from build123d import *

# Parameters (mm, degrees)
SKETCH_1_W          = 12
SKETCH_1_H          = 28
EXTRUDE_1_DEPTH     = 2
SKETCH_2_W          = 12
SKETCH_2_H          = 17
EXTRUDE_2_DEPTH     = 5
CUT_EXTRUDE_1_REACH = 18.031
SKETCH_3_R          = 1


with BuildPart() as part:
    # 草图1 → 凸台-拉伸1 (new body)
    with BuildSketch(Plane.XY):
        Rectangle(SKETCH_1_W, SKETCH_1_H)
    extrude(amount=-EXTRUDE_1_DEPTH)

    # 草图2 → 凸台-拉伸2 (add)
    with BuildSketch(Plane.XY):
        with Locations((0, 5.5)):
            Rectangle(SKETCH_2_W, SKETCH_2_H)
    extrude(amount=EXTRUDE_2_DEPTH)

    # 草图3 → 切除-拉伸1 (cut, up to next)
    with BuildSketch(Plane.XY, mode=Mode.PRIVATE) as cut_extrude_1_sk1:
        with Locations((0, -8)):
            Circle(SKETCH_3_R)
    cut_extrude_1_tool1 = extrude(cut_extrude_1_sk1.sketch, amount=-CUT_EXTRUDE_1_REACH, mode=Mode.PRIVATE) & part.part
    add(cut_extrude_1_tool1.solids().sort_by_distance((0, -8, 0))[0], mode=Mode.SUBTRACT)


solid = part.part
Here's how the part is built. I have some questions about the finished solid (model axes, mm). A direction names the side the tool comes from. Give positions to 0.01 mm unless a question says otherwise; leave off trailing zeros. Order: outer loops, then holes, each group sorted by start corner. A loop starts at its lowest first (then second) coordinate and runs counter-clockwise, first axis right, second up. Notation, with made-up numbers: (-6.75, -2) -> (49.25, -2) arc R16 cw to (49.25, 21) -> close; hole circle Ø11 at (26.5, 20). An arc over 180 degrees is marked (long way). Use a Markdown table: item, result. Add a question column.
Item 1: Imagine slicing it at B-B on x = 0. Please give me the cut outline in (y, z).
Item 2: Imagine slicing it at A-A on y = -8. Please give me the cut outline in (x, z), plus the area to 3 significant figures.
Item 3: Imagine slicing it at C-C on x = 4. Please give me the cut outline in (y, z).
Item 4: I need wall thicknesses on line 1 (Y direction, x = 0, z = -1); line 2 (Z direction, x = 3.25, y = -7.5); line 3 (Y direction, x = -3.75, z = 1.25). Which ranges of each line are inside material? Lowest first, please.
Item 5: Imagine slicing it at D-D on z = 2. Please give me the cut outline in (x, y).
Item 6: For faces 1 (the face through (0, -14, -1)), 2 (the face through (0, -10, 0)), which set-ups out of +Z, -Z, +X, -X, +Y, -Y let a thin tool reach every point of the face, with its end or its side?
Item 7: If we mould it in two halves opening along Y, with no side actions, what happens to faces 3 (the face through (0, 14, 1)), 4 (the face through (0, -3, 2)), 5 (the face through (0, 6, 5)), 6 (the face through (0, -7, -1))? For each: pulls with the +Y half, pulls with the -Y half, needs draft (parallel to the pull), parting line crosses it, or undercut.
Item 8: Will this pin go through, and if not, where does the flat tip stop? pin 1 (2 mm diameter, centred on x = 0.5, z = 1.5, fed in from -Y).
Data:
| question | item | result |
|---|---|---|
| 1 | outline | (-14, -2) -> (-9, -2) -> (-9, 0) -> (-14, 0) -> close; (-7, -2) -> (14, -2) -> (14, 5) -> (-3, 5) -> (-3, 0) -> (-7, 0) -> close |
| 2 | outline | (-6, -2) -> (-1, -2) -> (-1, 0) -> (-6, 0) -> close; (1, -2) -> (6, -2) -> (6, 0) -> (1, 0) -> close |
| 2 | area | 20.0 mm² |
| 3 | outline | (-14, -2) -> (14, -2) -> (14, 5) -> (-3, 5) -> (-3, 0) -> (-14, 0) -> close |
| 4 | line 1 | y = -14 to -9, -7 to 14 |
| 4 | line 2 | z = -2 to 0 |
| 4 | line 3 | y = -3 to 14 |
| 5 | outline | (-6, -3) -> (6, -3) -> (6, 14) -> (-6, 14) -> close |
| 6 | face 1 | +Z, -Z, +X, -X, -Y |
| 6 | face 2 | +Z, +X, -X, -Y |
| 7 | face 3 | pulls with the +Y half |
| 7 | face 4 | pulls with the -Y half |
| 7 | face 5 | needs draft |
| 7 | face 6 | undercut |
| 8 | pin 1 | stops at y = -3 |
